Geometry: final body of the model. Coordinates: model frame, mm. Face numbers are marked on the shaded views. A direction names the side the tool comes from. Give positions to 0.01 mm unless a question says otherwise; leave off trailing zeros. Loops run counter-clockwise (first coordinate to the right, second up) from the corner with the lowest first, then second, coordinate; pieces in that order, holes last. Notation, with made-up numbers: M 57,-12.75 L 101,-12.75 A12 ccw 101,-8.75 Z; hole C 47.5,41.5 d11. An arc over 180 degrees is marked long. One line per question, with ' | ' between items. Start each with the question number.
from build123d import *

# Parameters (mm, degrees)
F1_DEPTH = 12.7
F0_R     = 19.05
F2_DEPTH = 44.45
F4_DEPTH = 6.35


with BuildPart() as f1:
    # F0 (on Top) → F1 (new body)
    with BuildSketch(Plane.XY):
        with BuildLine():
            Line((-38.1, -25.4), (19.05, -25.4))
            ThreePointArc((19.05, -25.4), (6.35, 0), (19.05, 25.4))
            Line((19.05, 25.4), (-38.1, 25.4))
            Line((-38.1, 25.4), (-38.1, -25.4))
        make_face()
    extrude(amount=F1_DEPTH)

    # F0 (on Top) → F2 (join)
    with BuildSketch(Plane.XY):
        with BuildLine():
            ThreePointArc((19.05, 25.4), (6.35, 0), (19.05, -25.4))
            ThreePointArc((19.05, -25.4), (52.299032, -28.398063), (69.85, 0))
            ThreePointArc((69.85, 0), (52.299032, 28.398063), (19.05, 25.4))
        make_face()
        with Locations((38.1, 0)):
            Circle(F0_R, mode=Mode.SUBTRACT)
    extrude(amount=F2_DEPTH)

    # F3 (on Front) → F4 (join, symmetric)
    with BuildSketch(Plane.XZ):
        Polygon((6.35, 12.7), (19.05, 12.7), (19.05, 44.45), (6.35, 44.45), (-31.013487, 12.7), align=None)
    extrude(amount=F4_DEPTH, both=True)


solid = f1.part
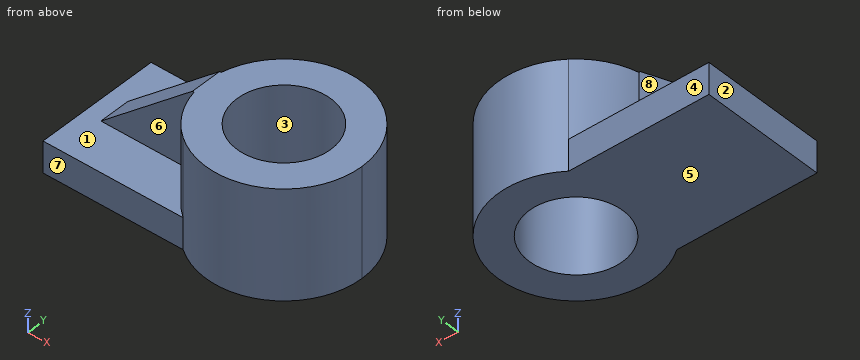
Q1. Material intervals for L1, parallel to Y at x = 38, z = 19; L2, parallel to Z at x = -13, y = -25; L3, parallel to X at y = 3, z = 3.5, sorted ascending.
Q2. Section C-C, the plane z = 21. Output: boundary loops of the cut face in (x, y).
Q3. Section B-B, the plane y = -9.5. Output: boundary loops of the cut face in (x, z), plus the area to 3 significant figures.
Q4. Section D-D, the plane x = -3. Output: boundary loops of the cut face in (y, z), plus the area to 3 significant figures.
Q5. Contact query for flat-ended pins moving along their axis: pin 1 (8 mm diameter, centred on x = 41.5, z = 27.5, fed in from +Y); pin 2 (10 mm diameter, centred on x = -17.5, z = 4.5, fed in from -Y); pin 3 (16 mm diameter, centred on x = -20.5, z = 21, fed in from +Y); pin 4 (4 mm diameter, centred on x = 15.5, y = 23, fed in from +Z). Output: stop coordinate, or through.
Q6. Draft query along X for the marked faces 1, 2 and 3. Return one class per face: released by +X, released by -X, zero draft, split by the parting line, or undercut.
Q7. Section A-A, the plane x = 38.1. Output: boundary loops of the cut face in (y, z).
Q8. Set-up query: the marked faces 4, 5, 6, 7 and 8. Return all of +Z, -Z, +X, -X, +Y, -Y with unobstructed straight access to the full face (end or side cutting, diameter ignored); none if empty.
Model answer:
1) L1: y = -31.75 to -19.05, 19.05 to 31.75 | L2: z = 0 to 12.7 | L3: x = -38.1 to 19.29, 56.91 to 69.71
2) outline: M -21.25,-6.35 L 6.99,-6.35 A31.75 ccw long 6.99,6.35 L -21.25,6.35 Z; hole C 38.1,0 d38.1
3) outline: M -38.1,0 L 21.59,0 L 21.59,44.45 L 7.8,44.45 L 7.8,12.7 L -38.1,12.7 Z; M 54.61,0 L 68.4,0 L 68.4,44.45 L 54.61,44.45 Z | area: 1,810 mm^2
4) outline: M -25.4,0 L 25.4,0 L 25.4,12.7 L 6.35,12.7 L 6.35,36.5 L -6.35,36.5 L -6.35,12.7 L -25.4,12.7 Z | area: 947 mm^2
5) pin 1: stops at y = 31.75 | pin 2: stops at y = -25.4 | pin 3: stops at y = 6.35 | pin 4: stops at z = 44.45
6) face 1: zero draft | face 2: released by -X | face 3: undercut
7) outline: M -31.75,0 L -19.05,0 L -19.05,44.45 L -31.75,44.45 Z; M 19.05,0 L 31.75,0 L 31.75,44.45 L 19.05,44.45 Z
8) face 4: +Z, -Z, -X, +Y | face 5: -Z, +X, -X, +Y, -Y | face 6: +Z, -X, -Y | face 7: +Z, -Z, -X, -Y | face 8: +Z, -X, +Y
